The listing builds one solid part. Answer for the finished solid, in the listing's coordinates (mm). Face numbers are marked on the shaded views. A direction names the side the tool comes from. Coordinates: 2 decimals unless noted, no trailing zeros. Loops run counter-clockwise (first coordinate to the right, second up) from the corner with the lowest first, then second, coordinate; pieces in that order, holes last. Notation, with made-up numbers: (31, -20.75) - (61, -20.75) arc R17 ccw to (61, -7.75) - close; hole circle Ø10 at (2.5, 17). An arc over 180 degrees is marked (long way). Return JSON: item names as keys, results as strings. Group by question number.
1. Section D-D (y = -226) is taken. Write down the section's boundary in (x, z).
2. Each of these flat-tipped pins is pushed along its axis until it touches: P1, Ø2, axis at y = -257.5, z = 24, coming from the +X side; P2, Ø2, axis at x = 28.5, z = -14.5, coming from the -Y side. Where does it stop, or does it pass through?
3. Section C-C (x = 111.5) is taken. Write down the section's boundary in (y, z).
4. The mould has two halves that part along Z. Classify the marked faces 4, 5, 6 and 7: pulls with the +Z half, pulls with the -Z half, needs draft (parallel to the pull), parting line crosses it, or undercut.
5. Which of the six approach directions +Z, -Z, +X, -X, +Y, -Y give full straight-line access (tool end or side, diameter ignored) to the marked faces 1, 2 and 3?
6. Section A-A (z = 48.5) is taken. Write down the section's boundary in (x, y), and give its area (3 significant figures).
7. Section B-B (y = -103.5) is taken. Write down the section's boundary in (x, z), and give its area (3 significant figures).
8. Find the intervals of material crossed by line 1 along Z through (x, y) = (-88, -41.5); line 2 along Y through (x, z) = (16, -28.5); line 3 along Y through (x, z) = (-113.5, 12), in increasing order.
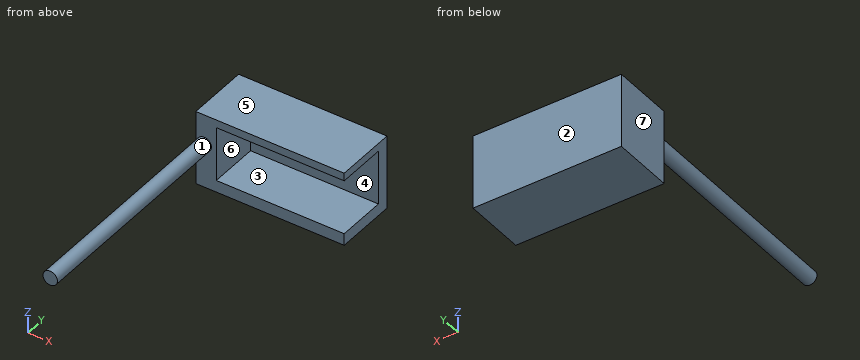
```python
from build123d import *

# Parameters (mm, degrees)
F0_W     = 304.8
F0_H     = 152.4
F1_DEPTH = 127
F2_W     = 262.756182
F2_H     = 111.728583
F3_DEPTH = 101.6
F4_R     = 14.821854
F5_DEPTH = 457.2


with BuildPart() as f1:
    # F0 (on Front) → F1 (new body)
    with BuildSketch(Plane.XZ):
        Rectangle(F0_W, F0_H)
    extrude(amount=F1_DEPTH)

    # F2 (on face) → F3 (cut, symmetric)
    with BuildSketch(Plane.XZ.offset(127)):
        with Locations((21.021909, 4.163234)):
            Rectangle(F2_W, F2_H)
    extrude(amount=F3_DEPTH, both=True, mode=Mode.SUBTRACT)

    # F4 (on face) → F5 (join)
    with BuildSketch(Plane.XZ.offset(127)):
        with Locations((-135.146677, 14.277183)):
            Circle(F4_R)
    extrude(amount=F5_DEPTH)


solid = f1.part
```
The answers:
{
 "1": {"outline": "circle Ø29.64 at (-135.15, 14.28)"},
 "2": {"P1": "stops at x = -123.16", "P2": "stops at y = -25.4"},
 "3": {"outline": "(-127, -76.2) - (0, -76.2) - (0, 76.2) - (-127, 76.2) - (-127, 60.03) - (-25.4, 60.03) - (-25.4, -51.7) - (-127, -51.7) - close"},
 "4": {"face 4": "undercut", "face 5": "pulls with the +Z half", "face 6": "undercut", "face 7": "needs draft"},
 "5": {"face 1": "-Y", "face 2": "+Z, -Z, +X, -X, +Y", "face 3": "+X, -Y"},
 "6": {"outline": "(-152.4, -127) - (-110.36, -127) - (-110.36, -25.4) - (152.4, -25.4) - (152.4, 0) - (-152.4, 0) - close", "area": "12,000 mm2"},
 "7": {"outline": "(-152.4, -76.2) - (152.4, -76.2) - (152.4, -51.7) - (-110.36, -51.7) - (-110.36, 60.03) - (152.4, 60.03) - (152.4, 76.2) - (-152.4, 76.2) - close", "area": "17,100 mm2"},
 "8": {"line 1": "z = -76.2 to -51.7, 60.03 to 76.2", "line 2": "y = -25.4 to 0", "line 3": "y = -127 to 0"}
}
